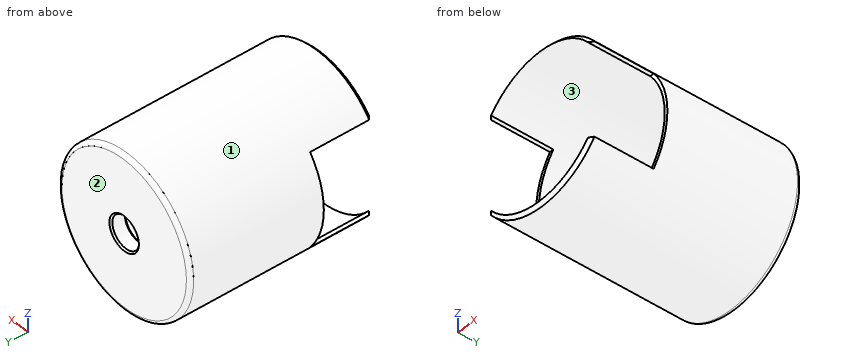
```python
from build123d import *

# Parameters (mm, degrees)
SKETCH_1_R               = 9.8
EXTRUDE_1_DEPTH          = 25
FILLET_1_R               = 0.5
SKETCH_5_R               = 9.4
CUT_EXTRUDE_2_DEPTH      = 23
CUT_EXTRUDE_3_DEPTH      = 29.584611279
CUT_EXTRUDE_3_DEPTH_BACK = 29.584611279
SKETCH_6_W               = 12
SKETCH_6_H               = 16
CHAMFER_4_SIZE           = 0.5
SKETCH_9_R               = 2
CUT_EXTRUDE_4_DEPTH      = 29.497192879
CHAMFER_5_SIZE           = 0.2


with BuildPart() as part:
    # 草图1 → 凸台-拉伸1 (new body)
    with BuildSketch(Plane(origin=(0, 0, 0), x_dir=(1, 0, 0), z_dir=(0, 1, 0))):
        with Locations(Location((0, 0, 0), (0, 0, 270))):
            Circle(SKETCH_1_R)
    extrude(amount=EXTRUDE_1_DEPTH)

    # 圆角1
    fillet_1_edges = [part.edges().sort_by_distance(p)[0] for p in [
        (0, 25, -9.8),
    ]]
    fillet(fillet_1_edges, radius=FILLET_1_R)

    # 草图5 → 切除-拉伸2 (cut)
    with BuildSketch(Plane.XZ):
        with Locations(Location((0, 0, 0), (0, 0, 270))):
            Circle(SKETCH_5_R)
    extrude(amount=-CUT_EXTRUDE_2_DEPTH, mode=Mode.SUBTRACT)

    # 草图6 → 切除-拉伸3 (cut, two sides: drawn at the far end of the back side and taken through both)
    with BuildSketch(Plane(origin=(0, 0, 0), x_dir=(0, 0, -1), z_dir=(1, 0, 0)).offset(-CUT_EXTRUDE_3_DEPTH_BACK)):
        Rectangle(SKETCH_6_W, SKETCH_6_H)
    extrude(amount=CUT_EXTRUDE_3_DEPTH + CUT_EXTRUDE_3_DEPTH_BACK, mode=Mode.SUBTRACT)

    # 倒角4
    # the kernel refuses this chamfer: 0.5 mm, written as the material it takes off along each edge
    with BuildSketch(Plane(origin=(0, 0, 0), x_dir=(0, 0, 1), z_dir=(-1, 0, 0))) as chamfer_4_piece_1:
        Polygon((9.8, CHAMFER_4_SIZE), (9.8 - CHAMFER_4_SIZE, 0), (9.8, 0), align=None)
    revolve(axis=Axis((0, 0, 0), (0, 1, 0)), revolution_arc=59.766699, mode=Mode.SUBTRACT)
    with BuildSketch(Plane(origin=(0, 0, 0), x_dir=(0.8640091314658966, 0, -0.5034761372136191), z_dir=(0.5034761372136191, 0, 0.8640091314658966))) as chamfer_4_piece_2:
        Polygon((9.8, CHAMFER_4_SIZE), (9.8 - CHAMFER_4_SIZE, 0), (9.8, 0), align=None)
    revolve(axis=Axis((0, 0, 0), (0, 1, 0)), revolution_arc=119.539505786, mode=Mode.SUBTRACT)
    with BuildSketch(Plane(origin=(0, 0, 0), x_dir=(-0.8639822947128161, 0, 0.503522188610171), z_dir=(-0.503522188610171, 0, -0.8639822947128161))) as chamfer_4_piece_3:
        Polygon((9.8, CHAMFER_4_SIZE), (9.8 - CHAMFER_4_SIZE, 0), (9.8, 0), align=None)
    revolve(axis=Axis((0, 0, 0), (0, 1, 0)), revolution_arc=59.766699, mode=Mode.SUBTRACT)

    # 草图9 → 切除-拉伸4 (cut, through all)
    with BuildSketch(Plane(origin=(0, 25, 0), x_dir=(1, 0, 0), z_dir=(0, 1, 0))):
        with Locations(Location((0, 0, 0), (0, 0, 270))):
            Circle(SKETCH_9_R)
    extrude(amount=-CUT_EXTRUDE_4_DEPTH, mode=Mode.SUBTRACT)

    # 倒角5
    chamfer_5_edges = [part.edges().sort_by_distance(p)[0] for p in [
        (0, 23, -2),
        (0, 25, -2),
    ]]
    chamfer(chamfer_5_edges, length=CHAMFER_5_SIZE)


solid = part.part
```
Model file for the job. Use its own axes, mm. Face numbers are marked on the shaded views. Coordinates: 2 decimals unless noted, no trailing zeros. Loops run counter-clockwise (first coordinate to the right, second up) from the corner with the lowest first, then second, coordinate; pieces in that order, holes last. Notation, with made-up numbers: M 68,68.25 L 84,68.25 A27 ccw 84,102.25 Z; hole C 42.5,-27.5 d4. An arc over 180 degrees is marked long. Use CSV: the item, a comma, the result in double quotes. Start each with the question number.
1. Two-plate mould, pull along Z, no slides. Class the marked faces 1, 2 and 3: pulls with the +Z half, pulls with the -Z half, needs draft (parallel to the pull), parting line crosses it, or undercut.
2. Flat gauge pin, fed straight in: pin 1 (4.5 mm diameter, centred on x = 0, z = 0, fed in from -Y). Where does the tip first touch, or does it go through?
3. Probe probe 1 along X at (y, z) = (23.95, 0); probe 2 along Y at (x, z) = (2.5, 7.25); probe 3 along Z at (x, y) = (0, 12.25). List the from-to ranges inside material, lowest first. Write a range as [from, to].
4. Band-saw the part on B-B, the plane y = 2. List the corners of the cut face in (x, z).
5. Band-saw the part on C-C, the plane y = 13. List the corners of the cut face in (x, z).
6. Band-saw the part on A-A, the plane z = 0. List the corners of the cut face in (x, y), then the cut area to 3 significant figures.
Entries:
1,face 1,"parting line crosses it"
1,face 2,"needs draft"
1,face 3,"undercut"
2,pin 1,"stops at y = 23"
3,probe 1,"x = [-9.8, -2], [2, 9.8]"
3,probe 2,"y = [23, 25]"
3,probe 3,"z = [-9.8, -9.4], [9.4, 9.8]"
4,outline,"M -7.75,-6 A9.8 ccw 7.75,-6 L 7.24,-6 A9.4 cw -7.24,-6 Z; M -7.75,6 L -7.24,6 A9.4 cw 7.24,6 L 7.75,6 A9.8 ccw Z"
5,outline,"C 0,0 d19.6; hole C 0,0 d18.8"
6,outline,"M -9.8,8 L -9.4,8 L -9.4,23 L -2.2,23 L -2,23.2 L -2,24.8 L -2.2,25 L -9.3,25 A0.5 ccw -9.8,24.5 Z; M 2,23.2 L 2.2,23 L 9.4,23 L 9.4,8 L 9.8,8 L 9.8,24.5 A0.5 ccw 9.3,25 L 2.2,25 L 2,24.8 Z"
6,area,"43.0 mm2"
